```python
from build123d import *

# Parameters (mm, degrees)
SKETCH1_W           = 93.98
SKETCH1_H           = 132.62918919
SKETCH1_R           = 2.54
SKETCH1_W_2         = 20.574
SKETCH1_H_2         = 16.002
SKETCH1_H_3         = 16.764
BOSS_EXTRUDE1_DEPTH = 5.08
BOSS_EXTRUDE2_DEPTH = 27.94
SKETCH4_W           = 22.098
SKETCH4_H           = 17.526
SKETCH4_H_2         = 18.288
BOSS_EXTRUDE3_DEPTH = 2.54


with BuildPart() as part:
    # Sketch1 → Boss-Extrude1 (new body)
    with BuildSketch(Plane.XY):
        Rectangle(SKETCH1_W, SKETCH1_H)
        with Locations((-14.224, -25.4)):
            Circle(SKETCH1_R, mode=Mode.SUBTRACT)
        with Locations((14.224, 25.4)):
            Circle(SKETCH1_R, mode=Mode.SUBTRACT)
        with Locations((29.337, 53.213)):
            Rectangle(SKETCH1_W_2, SKETCH1_H_2, mode=Mode.SUBTRACT)
        with Locations((-29.337, -52.578)):
            Rectangle(SKETCH1_W_2, SKETCH1_H_3, mode=Mode.SUBTRACT)
        with Locations((-29.337, 52.832)):
            Rectangle(SKETCH1_W_2, SKETCH1_H_3, mode=Mode.SUBTRACT)
        with Locations((29.337, -52.578)):
            Rectangle(SKETCH1_W_2, SKETCH1_H_3, mode=Mode.SUBTRACT)
        with BuildLine():
            Line((-33.02, -25.4), (-33.02, 25.4))
            ThreePointArc((-33.02, 25.4), (-29.21, 29.21), (-25.4, 25.4))
            Line((-25.4, 25.4), (-25.4, -25.4))
            ThreePointArc((-25.4, -25.4), (-29.21, -29.21), (-33.02, -25.4))
        make_face(mode=Mode.SUBTRACT)
        with BuildLine():
            Line((25.4, -25.4), (25.4, 25.4))
            ThreePointArc((25.4, 25.4), (29.21, 29.21), (33.02, 25.4))
            Line((33.02, 25.4), (33.02, -25.4))
            ThreePointArc((33.02, -25.4), (29.21, -29.21), (25.4, -25.4))
        make_face(mode=Mode.SUBTRACT)
    extrude(amount=BOSS_EXTRUDE1_DEPTH)

    # Sketch3 → Boss-Extrude2 (add)
    with BuildSketch(Plane(origin=(0, 0, 0), x_dir=(-1, 0, 0), z_dir=(0, 0, -1))):
        Polygon((-19.05, 45.212), (-39.624, 45.212), (-39.624, 61.214), (-41.148, 61.214), (-41.148, 43.688), (-19.05, 43.688), align=None)
        Polygon((19.05, 44.45), (39.624, 44.45), (39.624, 61.214), (41.148, 61.214), (41.148, 42.926), (19.05, 42.926), align=None)
        Polygon((19.05, -60.96), (39.624, -60.96), (39.624, -44.196), (41.148, -44.196), (41.148, -62.484), (19.05, -62.484), align=None)
        Polygon((-39.624, -44.196), (-39.624, -60.96), (-19.05, -60.96), (-19.05, -62.484), (-41.148, -62.484), (-41.148, -44.196), align=None)
    extrude(amount=BOSS_EXTRUDE2_DEPTH)

    # Sketch4 → Boss-Extrude3 (add)
    with BuildSketch(Plane(origin=(0, 0, -27.94), x_dir=(-1, 0, 0), z_dir=(0, 0, -1))):
        with Locations((-30.099, 52.451)):
            Rectangle(SKETCH4_W, SKETCH4_H)
        with Locations((30.099, 52.07)):
            Rectangle(SKETCH4_W, SKETCH4_H_2)
        with Locations((30.099, -53.34)):
            Rectangle(SKETCH4_W, SKETCH4_H_2)
        with Locations((-30.099, -53.34)):
            Rectangle(SKETCH4_W, SKETCH4_H_2)
    extrude(amount=-BOSS_EXTRUDE3_DEPTH)


solid = part.part
```
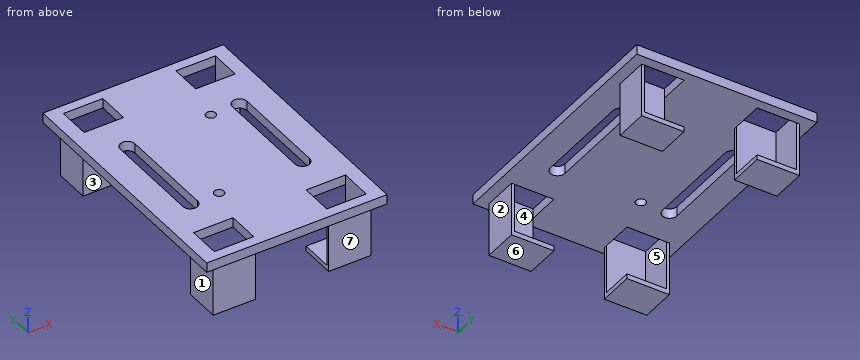
Can you work these out from the model? Positions are in its coordinate system, mm. Face numbers are marked on the shaded views. A direction names the side the tool comes from. Round coordinates to 2 decimals unless told otherwise and drop trailing zeros. Loops run counter-clockwise (first coordinate to the right, second up) from the corner with the lowest first, then second, coordinate; pieces in that order, holes last. Notation, with made-up numbers: M 50.25,29.5 L 67.25,29.5 A24 ccw 67.25,44.5 Z; hole C -1.5,73.5 d2. An arc over 180 degrees is marked long. Answer in a Markdown table with one row per item.
1. On a 3-axis mill with a long thin cutter (end or side, diameter ignored), from which of +Z, -Z, +X, -X, +Y, -Y can I reach the whole of each face in a straight line? I mean the marked faces 1, 2, 3 and 4. Say none if no direction works.
Established:
| item | result |
|---|---|
| face 1 | -Z, -X, +Y, -Y |
| face 2 | -Z, +X, +Y, -Y |
| face 3 | -Z, +X, -X |
| face 4 | +Z |
2. Thinking about a two-plate mould opening in Y: for the marked faces 5, 6 and 7, which applies, pulls with the +Y half, pulls with the -Y half, needs draft (parallel to the pull), parting line crosses it, or undercut?
Established:
| item | result |
|---|---|
| face 5 | undercut |
| face 6 | needs draft |
| face 7 | pulls with the -Y half |
3. If we section it at D-D, the plane y = -48: Please give me the cut outline in (x, z), plus the area to 3 significant figures.
Established:
| item | result |
|---|---|
| outline | M -46.99,0 L -41.15,0 L -41.15,-27.94 L -19.05,-27.94 L -19.05,-25.4 L -39.62,-25.4 L -39.62,5.08 L -46.99,5.08 Z; M -19.05,0 L 19.05,0 L 19.05,5.08 L -19.05,5.08 Z; M 19.05,-27.94 L 41.15,-27.94 L 41.15,0 L 46.99,0 L 46.99,5.08 L 39.62,5.08 L 39.62,-25.4 L 19.05,-25.4 Z |
| area | 458 mm² |
4. If we section it at C-C, the plane z = -23: Please give me the cut outline in (x, y), plus the area to 3 significant figures.
Established:
| item | result |
|---|---|
| outline | M -41.15,-62.48 L -19.05,-62.48 L -19.05,-60.96 L -39.62,-60.96 L -39.62,-44.2 L -41.15,-44.2 Z; M -41.15,42.93 L -19.05,42.93 L -19.05,44.45 L -39.62,44.45 L -39.62,61.21 L -41.15,61.21 Z; M 19.05,-62.48 L 41.15,-62.48 L 41.15,-44.2 L 39.62,-44.2 L 39.62,-60.96 L 19.05,-60.96 Z; M 19.05,43.69 L 41.15,43.69 L 41.15,61.21 L 39.62,61.21 L 39.62,45.21 L 19.05,45.21 Z |
| area | 236 mm² |
5. Please list where these lines run through material, in increasing order: line 1 (X direction, y = 25, z = 3); line 2 (X direction, y = -54, z = 2); line 3 (Y direction, x = 24.5, z = -8.5). Write a range as from..to.
Established:
| item | result |
|---|---|
| line 1 | -46.99..-33.02, -25.4..11.72, 16.73..25.4, 33.02..46.99 |
| line 2 | -46.99..-39.62, -19.05..19.05, 39.62..46.99 |
| line 3 | -62.48..-60.96, 43.69..45.21 |
6. If we section it at B-B, the plane x = -29.21: Please give me the cut outline in (y, z).
Established:
| item | result |
|---|---|
| outline | M -66.31,0 L -62.48,0 L -62.48,-27.94 L -44.2,-27.94 L -44.2,-25.4 L -60.96,-25.4 L -60.96,5.08 L -66.31,5.08 Z; M -44.2,0 L -29.21,0 L -29.21,5.08 L -44.2,5.08 Z; M 29.21,0 L 42.93,0 L 42.93,-27.94 L 61.21,-27.94 L 61.21,-25.4 L 44.45,-25.4 L 44.45,5.08 L 29.21,5.08 Z; M 61.21,0 L 66.31,0 L 66.31,5.08 L 61.21,5.08 Z |
7. I'm going to push flat-ended pins straight in: pin 1 Ø6.5 at (x, z) = (-30, -19) entering from +Y; pin 2 Ø5 at (y, z) = (-55, -4.5) entering from +X; pin 3 Ø5.5 at (y, z) = (-57, -13.5) entering from -X; pin 4 Ø12 at (x, z) = (13, -20) entering from +Y. Where does each tip first touch, or does it pass through?
Established:
| item | result |
|---|---|
| pin 1 | y = 44.45 |
| pin 2 | x = 41.15 |
| pin 3 | x = -41.15 |
| pin 4 | through |
8. If we section it at A-A, the plane y = -5: Please give me the cut outline in (x, z), plus the area to 3 significant figures.
Established:
| item | result |
|---|---|
| outline | M -46.99,0 L -33.02,0 L -33.02,5.08 L -46.99,5.08 Z; M -25.4,0 L 25.4,0 L 25.4,5.08 L -25.4,5.08 Z; M 33.02,0 L 46.99,0 L 46.99,5.08 L 33.02,5.08 Z |
| area | 400 mm² |
